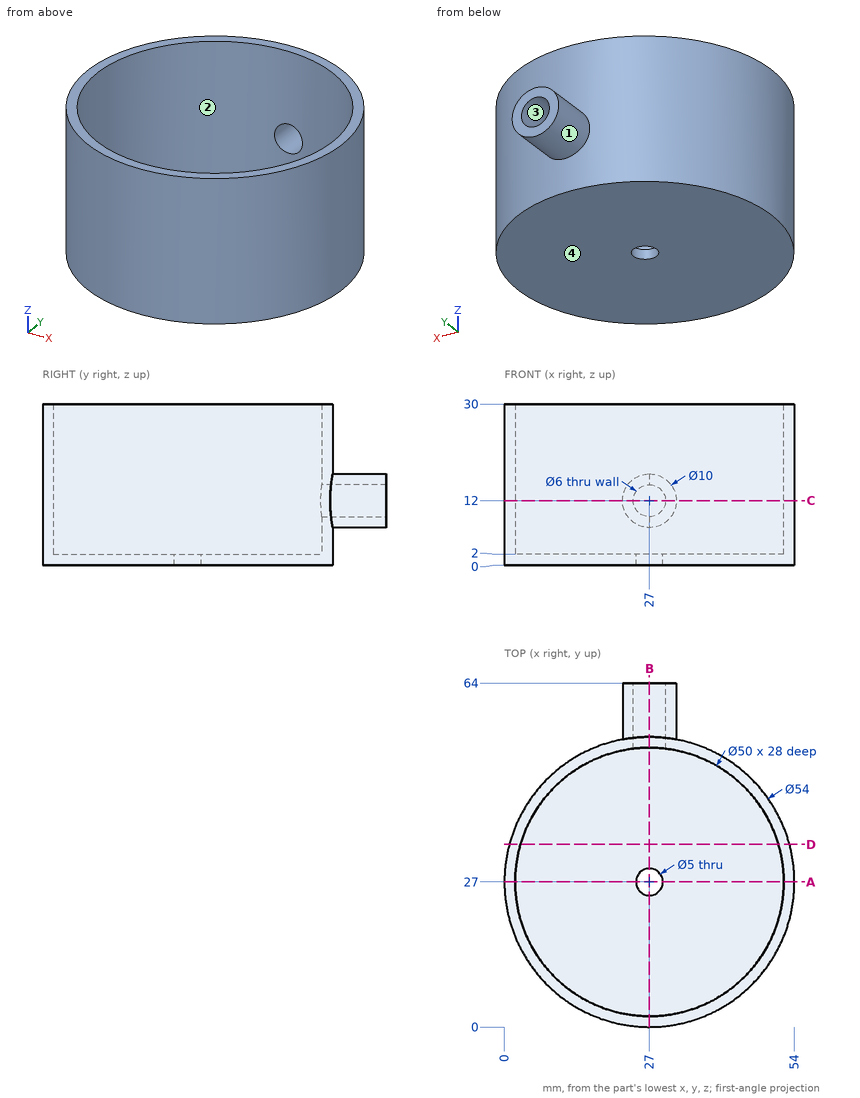
Can you work these out from the drawing? Everything is in mm from the part's minimum corner. Round coordinates to 2 decimals unless told otherwise and drop trailing zeros. Order: outer loops, then holes, each group sorted by start corner. A loop starts at its lowest first (then second) coordinate and runs counter-clockwise, first axis right, second up.
(1) If we section it at D-D (y = 34): Please give me the cut outline in (x, z).
Results are:
outline: (0.92, 0) - (53.08, 0) - (53.08, 30) - (51, 30) - (51, 2) - (3, 2) - (3, 30) - (0.92, 30) - close
(2) We'd pull the mould along X, two halves only. Please class the marked faces 1, 2, 3 and 4: +X half, -X half, draft (parallel to the pull), parting line (faces both ways), or undercut.
Results are:
face 1: parting line
face 2: undercut
face 3: undercut
face 4: draft
(3) If we section it at C-C (z = 12): Please give me the cut outline in (x, y), plus the area to 3 significant figures.
Results are:
outline: (22, 53.53) arc R27 ccw (long way) to (32, 53.53) - (32, 64) - (30, 64) - (30, 51.82) arc R25 cw (long way) to (24, 51.82) - (24, 64) - (22, 64) - close
area: 356 mm2
(4) If I drill on L1, parallel to Y at x = 27, z = 1.65; L2, parallel to Y at x = 19.5, z = 11; L3, parallel to X at y = 38, z = 8, over which ranges is the centre line in solid material (lowest first)?
Results are:
L1: y = 0 to 24.5, 29.5 to 54
L2: y = 1.06 to 3.15, 50.85 to 52.94
L3: x = 2.34 to 4.55, 49.45 to 51.66
(5) I'm going to push flat-ended pins straight in: pin 1 (25 mm diameter, centred on x = 24, y = 26, fed in from +Z); pin 2 (4 mm diameter, centred on y = 38, z = 15.5, fed in from -X); pin 3 (12 mm diameter, centred on x = 43.5, z = 20.5, fed in from +Y); pin 4 (10 mm diameter, centred on y = 24.5, z = 13.5, fed in from +X). Where does each tip first touch, or does it pass through?
Results are:
pin 1: stops at z = 2
pin 2: stops at x = 1.54
pin 3: stops at y = 51.87
pin 4: stops at x = 54
(6) If we section it at B-B (x = 27): Please give me the cut outline in (y, z), plus the area to 3 significant figures.
Results are:
outline: (0, 0) - (24.5, 0) - (24.5, 2) - (2, 2) - (2, 30) - (0, 30) - close; (29.5, 0) - (54, 0) - (54, 7) - (64, 7) - (64, 9) - (52, 9) - (52, 2) - (29.5, 2) - close; (52, 15) - (64, 15) - (64, 17) - (54, 17) - (54, 30) - (52, 30) - close
area: 238 mm2
(7) If we section it at A-A (y = 27): Please give me the cut outline in (x, z).
Results are:
outline: (0, 0) - (24.5, 0) - (24.5, 2) - (2, 2) - (2, 30) - (0, 30) - close; (29.5, 0) - (54, 0) - (54, 30) - (52, 30) - (52, 2) - (29.5, 2) - close
